Source: CAD feature listing. Evaluate the final solid. Frame: model axes, mm. A direction names the side the tool comes from. Give positions to 0.01 mm unless a question says otherwise; leave off trailing zeros. Loops run counter-clockwise (first coordinate to the right, second up) from the corner with the lowest first, then second, coordinate; pieces in that order, holes last. Notation, with made-up numbers: M 68,41.5 L 96,41.5 A10 cw 96,59.5 Z; hole C 55,68 d7. An arc over 180 degrees is marked long. Answer in a Markdown table with one row per item.
```python
from build123d import *

# Parameters (mm, degrees)
SKETCH1_W           = 20
SKETCH1_H           = 45
BOSS_EXTRUDE1_DEPTH = 17
CUT_EXTRUDE1_DEPTH  = 50.132473986
BOSS_EXTRUDE2_DEPTH = 5
SKETCH4_R           = 2
CUT_EXTRUDE2_DEPTH  = 53.096065111
SKETCH6_W           = 20
SKETCH6_H           = 20
BOSS_EXTRUDE3_DEPTH = 7
SKETCH8_W           = 8.2
SKETCH8_H           = 3.8
CUT_EXTRUDE3_DEPTH  = 45.522466239
CUT_EXTRUDE4_REACH  = 47.412
SKETCH7_R           = 2


with BuildPart() as part:
    # Sketch1 → Boss-Extrude1 (new body)
    with BuildSketch(Plane(origin=(0, 0, 0), x_dir=(1, 0, 0), z_dir=(0, 1, 0))):
        Rectangle(SKETCH1_W, SKETCH1_H)
    extrude(amount=BOSS_EXTRUDE1_DEPTH)

    # Sketch2 → Cut-Extrude1 (cut, through all)
    with BuildSketch(Plane.XY.offset(22.5)):
        with BuildLine():
            Line((0, 2), (-6.062177826, 5.5))
            ThreePointArc((-6.062177826, 5.5), (0, 16), (6.062177826, 5.5))
            Line((6.062177826, 5.5), (0, 2))
        make_face()
    extrude(amount=-CUT_EXTRUDE1_DEPTH, mode=Mode.SUBTRACT)

    # Sketch3 → Boss-Extrude2 (add)
    with BuildSketch(Plane.XY.offset(22.5)):
        Polygon((10, 0), (20, 0), (20, -10), (-20, -10), (-20, 0), (-10, 0), align=None)
    boss_extrude2 = extrude(amount=-BOSS_EXTRUDE2_DEPTH)

    # Mirror1: Boss-Extrude2 across plane
    add(boss_extrude2.mirror(Plane.XY))

    # Sketch4 → Cut-Extrude2 (cut, through all)
    with BuildSketch(Plane.XY.offset(22.5)):
        with Locations((16, -5)):
            Circle(SKETCH4_R)
        with Locations((-16, -5)):
            Circle(SKETCH4_R)
    extrude(amount=-CUT_EXTRUDE2_DEPTH, mode=Mode.SUBTRACT)

    # Sketch6 → Boss-Extrude3 (add)
    with BuildSketch(Plane(origin=(0, 17, 0), x_dir=(1, 0, 0), z_dir=(0, 1, 0))):
        Rectangle(SKETCH6_W, SKETCH6_H)
    extrude(amount=BOSS_EXTRUDE3_DEPTH)

    # Sketch8 → Cut-Extrude3 (cut, through all)
    with BuildSketch(Plane(origin=(10, 0, 0), x_dir=(0, 0, -1), z_dir=(1, 0, 0))):
        with Locations((0, 18.9)):
            Rectangle(SKETCH8_W, SKETCH8_H)
    extrude(amount=-CUT_EXTRUDE3_DEPTH, mode=Mode.SUBTRACT)

    # Sketch7 → Cut-Extrude4 (cut, up to next)
    with BuildSketch(Plane(origin=(0, 24, 0), x_dir=(1, 0, 0), z_dir=(0, 1, 0)), mode=Mode.PRIVATE) as cut_extrude4_sk1:
        with Locations(Location((0, 0, 0), (0, 0, 270))):
            Circle(SKETCH7_R)
    cut_extrude4_tool1 = extrude(cut_extrude4_sk1.sketch, amount=-CUT_EXTRUDE4_REACH, mode=Mode.PRIVATE) & part.part
    add(cut_extrude4_tool1.solids().sort_by_distance((0, 24, 0))[0], mode=Mode.SUBTRACT)


solid = part.part
```
Q1. Mould query, pull axis Y, two halves, no side actions, for faces 5 (the flat face through (2.4, 20.8, 0.1)), 6 (the flat face through (0, -10, 20)), 7 (the flat face through (20, -5, 20)). Classes: +Y half, -Y half, draft (parallel to the pull), parting line (faces both ways), or undercut.
Values follow:
| item | result |
|---|---|
| face 5 | undercut |
| face 6 | -Y half |
| face 7 | draft |
Q2. Contact query for flat-ended pins moving along their axis: pin 1 Ø5 at (x, z) = (3, 14.5) entering from +Y; pin 2 Ø22 at (x, z) = (1.5, -3) entering from -Y; pin 3 Ø4 at (x, y) = (1, 19.5) entering from +Z. Output: stop coordinate, or through.
Values follow:
| item | result |
|---|---|
| pin 1 | y = 17 |
| pin 2 | y = 0 |
| pin 3 | z = 10 |
Q3. Section query D-D (z = 7.5). Output: boundary loops of the cut face in (x, y).
Values follow:
| item | result |
|---|---|
| outline | M -10,0 L 10,0 L 10,24 L -10,24 Z; hole M -6.06,5.5 L 0,2 L 6.06,5.5 A7 ccw long Z |
Q4. Section query C-C (x = -16). Output: boundary loops of the cut face in (y, z), plus the area to 3 significant figures.
Values follow:
| item | result |
|---|---|
| outline | M -10,-22.5 L -7,-22.5 L -7,-17.5 L -10,-17.5 Z; M -10,17.5 L -7,17.5 L -7,22.5 L -10,22.5 Z; M -3,-22.5 L 0,-22.5 L 0,-17.5 L -3,-17.5 Z; M -3,17.5 L 0,17.5 L 0,22.5 L -3,22.5 Z |
| area | 60.0 mm^2 |
Q5. Section query A-A (z = 0). Output: boundary loops of the cut face in (x, y), plus the area to 3 significant figures.
Values follow:
| item | result |
|---|---|
| outline | M -10,0 L 10,0 L 10,17 L -10,17 Z; M -10,20.8 L -2,20.8 L -2,24 L -10,24 Z; M 2,20.8 L 10,20.8 L 10,24 L 2,24 Z; hole M -6.06,5.5 L 0,2 L 6.06,5.5 A7 ccw long Z |
| area | 246 mm^2 |
Q6. Reachability of faces 1 (the flat face through (0, 17, -16)), 2 (the flat face through (0, 17, 16)), 3 (the flat face through (0, 19, -4.1)), 4 (the flat face through (-15, 0, -20)) from +Z, -Z, +X, -X, +Y, -Y: full face, straight path, thin tool, end or side. Return the list, or none.
Values follow:
| item | result |
|---|---|
| face 1 | -Z, +X, -X, +Y |
| face 2 | +Z, +X, -X, +Y |
| face 3 | +X, -X |
| face 4 | +Z, -Z, -X, +Y |
Q7. Section query B-B (y = 9). Output: boundary loops of the cut face in (x, z).
Values follow:
| item | result |
|---|---|
| outline | M -10,-22.5 L -7,-22.5 L -7,22.5 L -10,22.5 Z; M 7,-22.5 L 10,-22.5 L 10,22.5 L 7,22.5 Z |
Q8. Ray query, probe 1 along X at (y, z) = (9, 13.5); probe 2 along X at (y, z) = (23, 0); probe 3 along Y at (x, z) = (16, 20). Return the intervals inside material, ascending. Write a range as from..to.
Values follow:
| item | result |
|---|---|
| probe 1 | -10..-7, 7..10 |
| probe 2 | -10..-2, 2..10 |
| probe 3 | -10..-7, -3..0 |
